```python
from build123d import *

# Parameters (mm, degrees)
SKETCH1_R           = 11.9
SKETCH1_R_2         = 1
SKETCH1_W           = 1.4
SKETCH1_H           = 4
BOSS_EXTRUDE1_DEPTH = 2


with BuildPart() as part:
    # Sketch1 → Boss-Extrude1 (new body)
    with BuildSketch(Plane.XY):
        with Locations((0.462805042, 1.624450899)):
            Circle(SKETCH1_R)
        with Locations((0.462805042, 1.624450899)):
            Circle(SKETCH1_R_2, mode=Mode.SUBTRACT)
        with Locations((10.462805042, 1.624450899)):
            Rectangle(SKETCH1_W, SKETCH1_H, mode=Mode.SUBTRACT)
        with Locations((-9.537194958, 1.624450899)):
            Rectangle(SKETCH1_W, SKETCH1_H, mode=Mode.SUBTRACT)
    extrude(amount=BOSS_EXTRUDE1_DEPTH)


solid = part.part
```
Verification items for the finished model (mm, model axes). A direction names the side the tool comes from. Coordinates: 2 decimals unless noted, no trailing zeros. Loops run counter-clockwise (first coordinate to the right, second up) from the corner with the lowest first, then second, coordinate; pieces in that order, holes last. Notation, with made-up numbers: (-17, 34.5) -> (-3, 34.5) arc R34 ccw to (-3, 67.5) -> close; hole circle Ø9 at (53, -21). An arc over 180 degrees is marked (long way). Put each result on its own line as item: value.
1. Tool access check on faces 4 (the face through (9.763, 2, 1)), 5 (the face through (0, -1, 0)). Record the directions out of +Z, -Z, +X, -X, +Y, -Y that give a thin tool (end or side, any length) a straight path to the whole face; none if there is none.
Result set:
face 4: +Z, -Z
face 5: -Z, +X, -X, +Y, -Y
2. Section check A-A, the plane x = 10.75. Record the boundary of the cut face in (y, z).
Result set:
outline: (-4.36, 0) -> (-0.38, 0) -> (-0.38, 2) -> (-4.36, 2) -> close; (3.62, 0) -> (7.61, 0) -> (7.61, 2) -> (3.62, 2) -> close
3. Section check B-B, the plane z = 0.3. Record the boundary of the cut face in (x, y).
Result set:
outline: circle Ø23.8 at (0.46, 1.62); hole (-10.24, -0.38) -> (-8.84, -0.38) -> (-8.84, 3.62) -> (-10.24, 3.62) -> close; hole circle Ø2 at (0.46, 1.62); hole (9.76, -0.38) -> (11.16, -0.38) -> (11.16, 3.62) -> (9.76, 3.62) -> close
4. Section check D-D, the plane y = -2.75. Record the boundary of the cut face in (x, z).
Result set:
outline: (-10.6, 0) -> (11.53, 0) -> (11.53, 2) -> (-10.6, 2) -> close
5. Thickness scan on line 1 (X direction, y = 0, z = 1.85); line 2 (X direction, y = -0.25, z = 1.45); line 3 (X direction, y = 0.75, z = 1.4). Record the ranges inside material, lowest first.
Result set:
line 1: x = -11.33 to -10.24, -8.84 to 9.76, 11.16 to 12.25
line 2: x = -11.29 to -10.24, -8.84 to 9.76, 11.16 to 12.21
line 3: x = -11.41 to -10.24, -8.84 to -0.02, 0.95 to 9.76, 11.16 to 12.33
6. Gauge pin test, flat ends, axial feed: P1, Ø1.1, axis at x = 10.5, z = 1, coming from the -Y side; P2, Ø0.7, axis at x = 11, z = 1, coming from the +Y side. Record the tip position at first contact, or that the pin passes through.
Result set:
P1: stops at y = -5.56
P2: stops at y = 7.78
7. Mould release check, pull along X, two halves, no side actions. Record for faces 1 (the face through (-8.98, -5.62, 0.99)), 2 (the face through (0, -1, 2)), 3 (the face through (11.163, 2, 1)): pulls with the +X half, pulls with the -X half, needs draft (parallel to the pull), parting line crosses it, or undercut.
Result set:
face 1: parting line crosses it
face 2: needs draft
face 3: undercut
8. Section check C-C, the plane x = 0.5. Record the boundary of the cut face in (y, z).
Result set:
outline: (-10.28, 0) -> (0.63, 0) -> (0.63, 2) -> (-10.28, 2) -> close; (2.62, 0) -> (13.52, 0) -> (13.52, 2) -> (2.62, 2) -> close
